Verification items for the finished model (mm, model axes). Face numbers are marked on the shaded views. A direction names the side the tool comes from. Coordinates: 2 decimals unless noted, no trailing zeros. Write each loop counter-clockwise with the first axis right and the second up, starting at its lowest first coordinate (ties: lowest second). Pieces come first, ordered by that corner, then holes. Notation, with made-up numbers: (10, 88) -> (23, 88) arc R27 cw to (23, 112) -> close; hole circle Ø6 at (58.25, 11.5). An arc over 180 degrees is marked (long way). Answer in a Markdown table with one row per item.
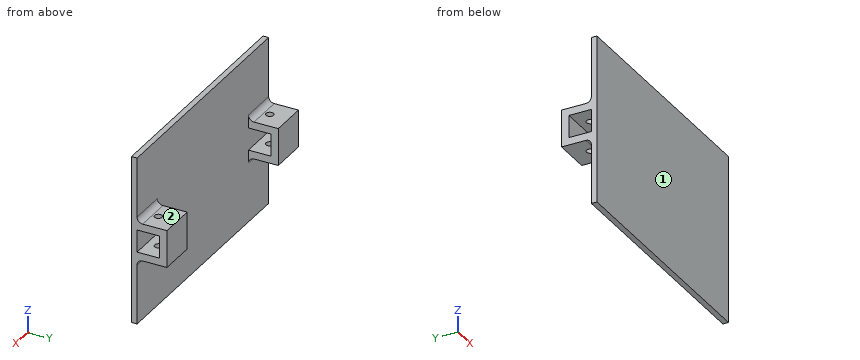
Autodesk Fusion 360 part; units mm, degrees
sketch "Sketch1" plane through (0, 0, 0) normal (0, 1, 0) x (1, 0, 0)
  line L0 (-50, 5) -> (15, 5)
  line L1 (15, 5) -> (15, -40)
  line L2 (15, -40) -> (-50, -40)
  line L3 (-50, -40) -> (-50, 5)
  dimension "d1" = 65
  dimension "d2" = 45
extrude "Extrude1" add sketch "Sketch1" along normal blind 2
sketch "Sketch2" plane through (0, 2, 0) normal (0, 1, 0) x (-1, 0, 0)
  line L0 (50, 40) -> (-15, 40)
  line L1 (-15, 40) -> (-15, -5)
  line L2 (-15, -5) -> (50, -5)
  line L3 (50, -5) -> (50, 40)
  line L4 (50, 17.5) -> (-15, 17.5)
  line L5 (50, 14.5) -> (-15, 14.5)
  line L6 (-15, 20.5) -> (50, 20.5)
  line L7 (50, 12.5) -> (-15, 12.5)
  line L8 (-15, 22.5) -> (50, 22.5)
  line L9 (50, 17.5) -> (40, 17.5)
  line L10 (40, 17.5) -> (40, 12.5)
  line L11 (40, 17.5) -> (40, 22.5)
  line L12 (-15, 17.5) -> (-5, 17.5)
  line L13 (-5, 17.5) -> (-5, 12.5)
  line L14 (-5, 17.5) -> (-5, 22.5)
  dimension "d5" = 3
  dimension "d6" = 6
  dimension "d7" = -2
  dimension "d8" = -2
  dimension "d9" = 10
  dimension "d15" = 10
extrude "Extrude2" add sketch "Sketch2" along normal blind 7 contours L3 L6 L8 L11 | L3 L5 L7 L10
sketch "Sketch3" plane through (0, 0, 14.5) normal (0, 0, 1) x (1, 0, 0)
  line L0 (-50, 2) -> (-40, 2)
  line L1 (-40, 2) -> (-40, 9)
  line L2 (-40, 9) -> (-50, 9)
  line L3 (-50, 9) -> (-50, 2)
  line L4 (-40, 8) -> (-50, 8)
  dimension "d12" = -1
extrude "Extrude4" add sketch "Sketch2" along normal blind 7 contours L1 L6 L8 L14 | L1 L5 L7 L13
sketch "Sketch4" plane through (0, 0, 14.5) normal (0, 0, 1) x (1, 0, 0)
  line L0 (5, 2) -> (15, 2)
  line L1 (15, 2) -> (15, 9)
  line L2 (15, 9) -> (5, 9)
  line L3 (5, 9) -> (5, 2)
  line L4 (15, 8) -> (5, 8)
  dimension "d18" = -1
extrude "Extrude5" add sketch "Sketch4" along normal blind 6 contours L1 L2 L3 L4
extrude "Extrude6" add 1 faces at (8.3333, 9, 19.1667) along direction (0, 1, 0) blind 1
extrude "Extrude7" add sketch "Sketch3" along normal blind 1 contours L1 L2 L3 L4
extrude "Extrude8" add 1 faces at (-46.6667, 8.6667, 15.5) along direction (0, 0, 1) blind 5
extrude "Extrude9" add 1 faces at (-43.3333, 9, 15.8333) along direction (0, 1, 0) blind 1
extrude "Extrude10" cut 1 faces at (-28.3333, 0, 10) along direction (0, 1, 0) blind 0.5
sketch "Sketch5" plane through (0, 0, 22.5) normal (0, 0, 1) x (1, 0, 0)
  line L0 (-50, 2) -> (-40, 2)
  line L1 (-40, 2) -> (-40, 10)
  line L2 (-40, 10) -> (-50, 10)
  line L3 (-50, 10) -> (-50, 2)
  line L4 (-50, 2) -> (-50, 2.3478)
  circle A0 centre (-45, 5) radius 1
  dimension "d31" = 2
hole "Hole1" at (-45, 5, 22.5) direction (0, 0, -1) diameter 2 depth 2 tip angle 180
sketch "Sketch6" plane through (0, 0, 12.5) normal (0, 0, -1) x (-1, 0, 0)
  line L0 (40, 2) -> (50, 2)
  line L1 (50, 2) -> (50, 10)
  line L2 (50, 10) -> (40, 10)
  line L3 (40, 10) -> (40, 2)
  line L4 (40, 2) -> (45, 2)
  line L5 (45, 2) -> (45, 5)
  circle A0 centre (45, 5) radius 1
  dimension "d35" = 3
  dimension "d36" = 2
hole "Hole2" at (-45, 5, 12.5) direction (0, 0, 1) diameter 2 depth 2 tip angle 180
sketch "Sketch7" plane through (0, 0, 12.5) normal (0, 0, -1) x (-1, 0, 0)
  line L0 (-15, 2) -> (-5, 2)
  line L1 (-5, 2) -> (-5, 10)
  line L2 (-5, 10) -> (-15, 10)
  line L3 (-15, 10) -> (-15, 2)
  line L4 (-15, 2) -> (-10, 2)
  line L5 (-10, 2) -> (-10, 5)
  circle A0 centre (-10, 5) radius 1
  dimension "d40" = 3
  dimension "d41" = 2
hole "Hole3" at (10, 5, 12.5) direction (0, 0, 1) diameter 2 depth 2 tip angle 180
sketch "Sketch8" plane through (0, 2, 0) normal (0, 1, 0) x (-1, 0, 0)
sketch "Sketch9" plane through (0, 0, 22.5) normal (0, 0, 1) x (1, 0, 0)
  line L0 (5, 2) -> (15, 2)
  line L1 (15, 2) -> (15, 10)
  line L2 (15, 10) -> (5, 10)
  line L3 (5, 10) -> (5, 2)
  line L4 (5, 2) -> (10, 2)
  line L5 (10, 2) -> (10, 5)
  circle A0 centre (10, 5) radius 1
  dimension "d45" = 3
  dimension "d46" = 2
hole "Hole4" at (10, 5, 22.5) direction (0, 0, -1) diameter 2 depth 2 tip angle 180
fillet "Fillet1" radius 1.5 4 edges at (-45, 2, 12.5) (-45, 2, 22.5) (10, 2, 22.5) (10, 2, 12.5)
extrude "Extrude3" add sketch "Sketch3" along normal blind 6 contours L1 L2 L3 L4
1. Section check B-B, the plane y = 5. State how many separate pieces and enclosed holes the cut face has, plus the area to 3 significant figures.
Geometry says:
| item | result |
|---|---|
| separate pieces | 8 |
| enclosed holes | 0 |
| area | 64.0 mm^2 |
2. Section check C-C, the plane x = -45. Record the boundary of the cut face in (y, z), plus the area to 3 significant figures.
Geometry says:
| item | result |
|---|---|
| outline | (0.5, -5) -> (2, -5) -> (2, 11) arc R1.5 cw to (3.5, 12.5) -> (4, 12.5) -> (4, 14.5) -> (2, 14.5) -> (2, 20.5) -> (4, 20.5) -> (4, 22.5) -> (3.5, 22.5) arc R1.5 cw to (2, 24) -> (2, 40) -> (0.5, 40) -> close; (6, 12.5) -> (10, 12.5) -> (10, 22.5) -> (6, 22.5) -> (6, 20.5) -> (8, 20.5) -> (8, 14.5) -> (6, 14.5) -> close |
| area | 104 mm^2 |
3. Tool access check on the marked faces 1 and 2. Record the directions out of +Z, -Z, +X, -X, +Y, -Y that give a thin tool (end or side, any length) a straight path to the whole face; none if there is none.
Geometry says:
| item | result |
|---|---|
| face 1 | +Z, -Z, +X, -X, -Y |
| face 2 | +Z, +X, -X, +Y |
4. Section check D-D, the plane z = 28.5. Record the boundary of the cut face in (x, y).
Geometry says:
| item | result |
|---|---|
| outline | (-50, 0.5) -> (15, 0.5) -> (15, 2) -> (-50, 2) -> close |
5. Section check A-A, the plane x = 8. Record the boundary of the cut face in (y, z).
Geometry says:
| item | result |
|---|---|
| outline | (0.5, -5) -> (2, -5) -> (2, 11) arc R1.5 cw to (3.5, 12.5) -> (10, 12.5) -> (10, 22.5) -> (3.5, 22.5) arc R1.5 cw to (2, 24) -> (2, 40) -> (0.5, 40) -> close; hole (2, 14.5) -> (8, 14.5) -> (8, 20.5) -> (2, 20.5) -> close |
6. Thickness scan on line 1 (X direction, y = 5, z = 21.95); line 2 (Z direction, x = 12, y = 7.75); line 3 (Y direction, x = -45.5, z = 19.5). Record the ranges inside material, lowest first. Write a range as from..to.
Geometry says:
| item | result |
|---|---|
| line 1 | -50..-46, -44..-40, 5..9, 11..15 |
| line 2 | 12.5..14.5, 20.5..22.5 |
| line 3 | 0.5..2, 8..10 |
7. Depth check by flat-ended pin: P1, Ø1.5, axis at x = -24, y = 4.5, coming from the +Z side; P2, Ø5, axis at x = -39, y = 9, coming from the +Z side; P3, Ø5, axis at x = 11, y = 3.5, coming from the +Z side; P4, Ø5, axis at x = 8, y = 5.5, coming from the -Z side. Enter the tip coordinate at first touch or a pass-through.
Geometry says:
| item | result |
|---|---|
| P1 | through |
| P2 | z = 22.5 |
| P3 | z = 40 |
| P4 | z = 12.41 |
